The figure shows three views and two pictorial views of one solid part (mm, origin at its lowest corner). Answer the questions. Round coordinates to 2 decimals unless told otherwise and drop trailing zeros. Write each loop counter-clockwise with the first axis right and the second up, starting at its lowest first coordinate (ties: lowest second). Pieces come first, ordered by that corner, then holes.
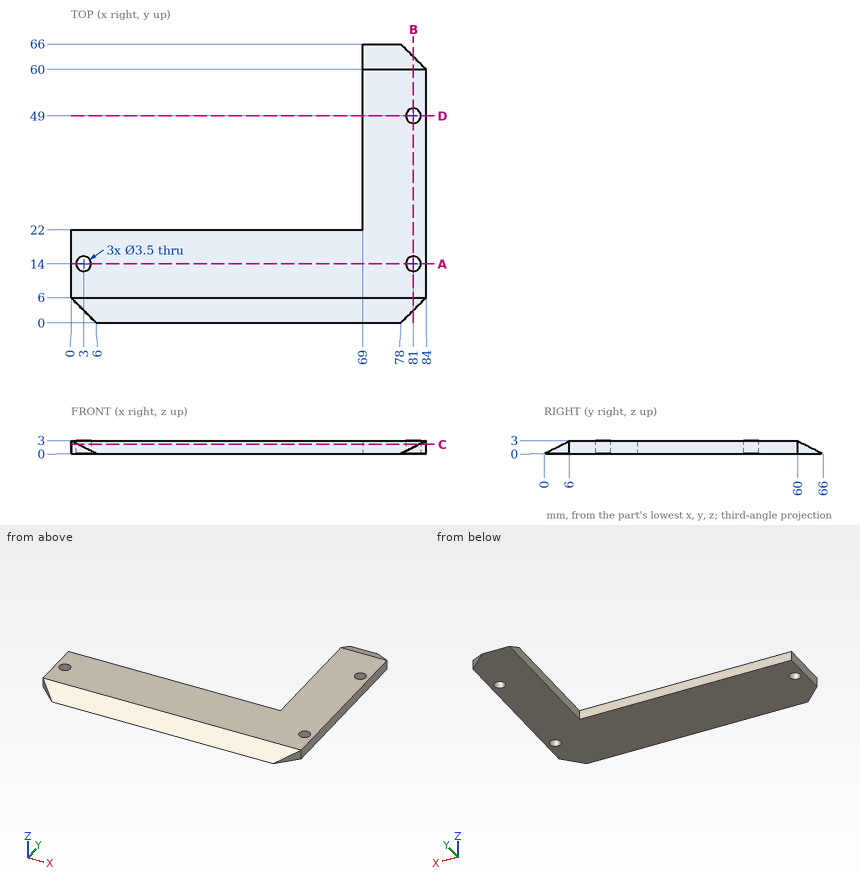
Q1. Section D-D (y = 49) is taken. Determine the outline of the cut face in (x, z), then the cut area to 3 significant figures.
Verdict:
outline: (69, 0) - (79.25, 0) - (79.25, 3) - (69, 3) - close; (82.75, 0) - (84, 0) - (84, 3) - (82.75, 3) - close
area: 34.5 mm2
Q2. Flat-ended cylindrical pins translate along their axes: pin 1 Ø4.5 at (x, y) = (81, 49) entering from +Z; pin 2 Ø1.5 at (y, z) = (28, 2.5) entering from -X. Find the tip coordinate at first contact, or state that the pin passes through.
Verdict:
pin 1: stops at z = 3
pin 2: stops at x = 69
Q3. Section C-C (z = 2.2) is taken. Determine the outline of the cut face in (x, y), then the cut area to 3 significant figures.
Verdict:
outline: (0, 6) - (1.6, 4.4) - (82.4, 4.4) - (84, 6) - (84, 60) - (82.4, 61.6) - (69, 61.6) - (69, 22) - (0, 22) - close; hole circle Ø3.5 at (3, 14); hole circle Ø3.5 at (81, 14); hole circle Ø3.5 at (81, 49)
area: 2,040 mm2
Q4. Straight lines are drawn through the part: probe 1 along X at (y, z) = (15.5, 0.9); probe 2 along Y at (x, z) = (81, 2.35); probe 3 along X at (y, z) = (26, 1.75). For each, find the intervals that lie inside material, in ascending order.
Verdict:
probe 1: x = 0 to 2.1, 3.9 to 80.1, 81.9 to 84
probe 2: y = 4.7 to 12.25, 15.75 to 47.25, 50.75 to 61.3
probe 3: x = 69 to 84
Q5. Section A-A (y = 14) is taken. Determine the outline of the cut face in (x, z).
Verdict:
outline: (0, 0) - (1.25, 0) - (1.25, 3) - (0, 3) - close; (4.75, 0) - (79.25, 0) - (79.25, 3) - (4.75, 3) - close; (82.75, 0) - (84, 0) - (84, 3) - (82.75, 3) - close
Q6. Section B-B (x = 81) is taken. Determine the outline of the cut face in (y, z), then the cut area to 4 significant figures.
Verdict:
outline: (3, 0) - (12.25, 0) - (12.25, 3) - (6, 3) - (3, 1.5) - close; (15.75, 0) - (47.25, 0) - (47.25, 3) - (15.75, 3) - close; (50.75, 0) - (63, 0) - (63, 1.5) - (60, 3) - (50.75, 3) - close
area: 154.5 mm2
